Model file for the job. Use its own axes, mm. A direction names the side the tool comes from. Give positions to 0.01 mm unless a question says otherwise; leave off trailing zeros. Loops run counter-clockwise (first coordinate to the right, second up) from the corner with the lowest first, then second, coordinate; pieces in that order, holes last. Notation, with made-up numbers: M 88,39.25 L 112,39.25 A33 ccw 112,71.25 Z; hole C -4.75,-4 d6. An arc over 180 degrees is marked long. Answer in a Markdown table with one row per item.
```python
from build123d import *

# Parameters (mm, degrees)
BOSS_EXTRUDE1_DEPTH = 1.6
SKETCH2_R           = 0.762
CUT_EXTRUDE1_DEPTH  = 2.6


with BuildPart() as part:
    # Sketch1 → Boss-Extrude1 (new body)
    with BuildSketch(Plane.XY):
        with BuildLine():
            Line((-35.56, 25.4), (35.56, 25.4))
            Line((35.56, 25.4), (35.56, 28.702))
            ThreePointArc((35.56, 28.702), (38.1, 31.242), (40.64, 28.702))
            Line((40.64, 28.702), (40.64, -28.702))
            ThreePointArc((40.64, -28.702), (38.1, -31.242), (35.56, -28.702))
            Line((35.56, -28.702), (35.56, -25.4))
            Line((35.56, -25.4), (-35.56, -25.4))
            Line((-35.56, -25.4), (-35.56, -28.702))
            ThreePointArc((-35.56, -28.702), (-38.1, -31.242), (-40.64, -28.702))
            Line((-40.64, -28.702), (-40.64, 28.702))
            ThreePointArc((-40.64, 28.702), (-38.1, 31.242), (-35.56, 28.702))
            Line((-35.56, 28.702), (-35.56, 25.4))
        make_face()
    extrude(amount=BOSS_EXTRUDE1_DEPTH)

    # Sketch2 → Cut-Extrude1 (cut, through all)
    with BuildSketch(Plane.XY.offset(1.6)):
        with Locations((38.1, 28.702)):
            Circle(SKETCH2_R)
        with Locations((-38.1, 28.702)):
            Circle(SKETCH2_R)
        with Locations((38.1, -28.702)):
            Circle(SKETCH2_R)
        with Locations((-38.1, -28.702)):
            Circle(SKETCH2_R)
    extrude(amount=-CUT_EXTRUDE1_DEPTH, mode=Mode.SUBTRACT)


solid = part.part
```
(1) Wall check: L1, parallel to Y at x = 38.1, z = 0.95; L2, parallel to X at y = -26.5, z = 1.4; L3, parallel to Y at x = -30, z = 1.2. Give the ranges that are in metal, low to high.
Established:
| item | result |
|---|---|
| L1 | y = -31.24 to -29.46, -27.94 to 27.94, 29.46 to 31.24 |
| L2 | x = -40.64 to -35.56, 35.56 to 40.64 |
| L3 | y = -25.4 to 25.4 |
(2) Saw through at B-B, the plane x = 8.5. Give the cut face in (y, z).
Established:
| item | result |
|---|---|
| outline | M -25.4,0 L 25.4,0 L 25.4,1.6 L -25.4,1.6 Z |
(3) Flat gauge pins, fed straight in: P1, Ø0.5, axis at x = 11, z = 1, coming from the -Y side; P2, Ø0.9, axis at x = 38.1, y = 28.702, coming from the -Z side; P3, Ø0.5, axis at x = 7, z = 0.5, coming from the +Y side. Where does each tip first touch, or does it go through?
Established:
| item | result |
|---|---|
| P1 | stops at y = -25.4 |
| P2 | passes through |
| P3 | stops at y = 25.4 |
(4) Mould opens along X. For faces 1 (the flat face through (40.64, 0, 1)), 2 (the flat face through (-35.56, 27, 1)), 3 (the flat face through (1, 0, 0)), 4 (the cylindrical face through (38.16, -31.24, 0.79)) say: pulls with the +X half, pulls with the -X half, needs draft (parallel to the pull), parting line crosses it, or undercut.
Established:
| item | result |
|---|---|
| face 1 | pulls with the +X half |
| face 2 | undercut |
| face 3 | needs draft |
| face 4 | undercut |
(5) Which spindle directions (+Z, -Z, +X, -X, +Y, -Y) get a long thin tool onto all of the face, cutting with end or side? Do faces 5 (the flat face through (-40.64, 0, 1)), 6 (the flat face through (-35.56, -27, 1)), 7 (the flat face through (0, 25.4, 1)). Say none if no direction does.
Established:
| item | result |
|---|---|
| face 5 | +Z, -Z, -X, +Y, -Y |
| face 6 | +Z, -Z, -Y |
| face 7 | +Z, -Z, +Y |
(6) Saw through at A-A, the plane z = 1.1. Give the cut face in (x, y).
Established:
| item | result |
|---|---|
| outline | M -40.64,-28.7 A2.54 ccw -35.56,-28.7 L -35.56,-25.4 L 35.56,-25.4 L 35.56,-28.7 A2.54 ccw 40.64,-28.7 L 40.64,28.7 A2.54 ccw 35.56,28.7 L 35.56,25.4 L -35.56,25.4 L -35.56,28.7 A2.54 ccw -40.64,28.7 Z; hole C -38.1,-28.7 d1.52; hole C -38.1,28.7 d1.52; hole C 38.1,-28.7 d1.52; hole C 38.1,28.7 d1.52 |
